Here's how the part is built. I have some questions about the finished solid (model axes, mm). Coordinates: 2 decimals unless noted, no trailing zeros. Order: outer loops, then holes, each group sorted by start corner. A loop starts at its lowest first (then second) coordinate and runs counter-clockwise, first axis right, second up. Notation, with made-up numbers: M 55.25,27 L 83.25,27 A19 ccw 83.25,52 Z; hole C -3.5,11 d2. An arc over 180 degrees is marked long. Answer as CSV lines item,"result". Start each with the question number.
```python
from build123d import *

# Parameters (mm, degrees)
ESQUISSE1_W        = 420
ESQUISSE1_H        = 560
ESQUISSE1_R        = 6.1
ESQUISSE1_R_2      = 7.5
BOSS_EXTRU_1_DEPTH = 12


with BuildPart() as part:
    # Esquisse1 → Boss.-Extru.1 (new body)
    with BuildSketch(Plane(origin=(0, 0, 0), x_dir=(1, 0, 0), z_dir=(0, 1, 0))):
        with Locations((0, -70)):
            Rectangle(ESQUISSE1_W, ESQUISSE1_H)
        with Locations(Location((-63.273726515, 173.843134845, 0), (0, 0, 270))):  # turned: the seam where the file's is
            Circle(ESQUISSE1_R, mode=Mode.SUBTRACT)
        with Locations(Location((-175, -61.5, 0), (0, 0, 270))):  # turned: the seam where the file's is
            Circle(ESQUISSE1_R_2, mode=Mode.SUBTRACT)
        with Locations(Location((110.0032143, -211.5, 0), (0, 0, 270))):  # turned: the seam where the file's is
            Circle(ESQUISSE1_R_2, mode=Mode.SUBTRACT)
        with Locations(Location((175, -61.5, 0), (0, 0, 270))):  # turned: the seam where the file's is
            Circle(ESQUISSE1_R_2, mode=Mode.SUBTRACT)
        with Locations(Location((185, 0, 0), (0, 0, 270))):  # turned: the seam where the file's is
            Circle(ESQUISSE1_R, mode=Mode.SUBTRACT)
        with Locations(Location((-109.9967857, -211.5, 0), (0, 0, 270))):  # turned: the seam where the file's is
            Circle(ESQUISSE1_R_2, mode=Mode.SUBTRACT)
        with Locations(Location((151.543128193, 106.111640725, 0), (0, 0, 90))):  # turned: the seam where the file's is
            Circle(ESQUISSE1_R, mode=Mode.SUBTRACT)
        with Locations(Location((-151.543128193, 106.111640725, 0), (0, 0, 270))):  # turned: the seam where the file's is
            Circle(ESQUISSE1_R, mode=Mode.SUBTRACT)
        with Locations(Location((-185, 0, 0), (0, 0, 90))):  # turned: the seam where the file's is
            Circle(ESQUISSE1_R, mode=Mode.SUBTRACT)
        with Locations(Location((63.273726515, 173.843134845, 0), (0, 0, 90))):  # turned: the seam where the file's is
            Circle(ESQUISSE1_R, mode=Mode.SUBTRACT)
        with Locations(Location((-145.781989417, -113.897372935, 0), (0, 0, 270))):  # turned: the seam where the file's is
            Circle(ESQUISSE1_R, mode=Mode.SUBTRACT)
        with Locations(Location((-78.184378422, -167.666940602, 0), (0, 0, 270))):  # turned: the seam where the file's is
            Circle(ESQUISSE1_R, mode=Mode.SUBTRACT)
        with Locations(Location((145.781989417, -113.897372935, 0), (0, 0, 90))):  # turned: the seam where the file's is
            Circle(ESQUISSE1_R, mode=Mode.SUBTRACT)
        with Locations(Location((78.184378422, -167.666940602, 0), (0, 0, 90))):  # turned: the seam where the file's is
            Circle(ESQUISSE1_R, mode=Mode.SUBTRACT)
        with BuildLine():
            Line((10.5, 164.654013459), (10.5, 159.154013459))
            ThreePointArc((10.5, 159.154013459), (0, -159.5), (-10.5, 159.154013459))
            Line((-10.5, 159.154013459), (-10.5, 164.654013459))
            Line((-10.5, 164.654013459), (10.5, 164.654013459))
        make_face(mode=Mode.SUBTRACT)
    extrude(amount=BOSS_EXTRU_1_DEPTH)


solid = part.part
```
1) Suppose I cut it at C-C on z = 0. Please give me the cut outline in (x, y), plus the area to 3 significant figures.
2) If we mould it in two halves opening along Z, with no side actions, what happens to faces 1 (the face through (-3, 6, 350)), 2 (the face through (145.51, 5.92, 119.99)), 3 (the face through (-3, 0, 191))? For each: released by +Z, released by -Z, zero draft, split by the parting line, or undercut.
3) Suppose I cut it at B-B on x = 0. Please give me the cut outline in (y, z), plus the area to 3 significant figures.
4) Suppose I cut it at A-A on z = 211.5. Please give me the cut outline in (x, y), plus the area to 3 significant figures.
5) I need wall thicknesses on line 1 (X direction, y = 6.25, z = 211.5); line 2 (X direction, y = 4.75, z = -178); line 3 (Z direction, x = 0, y = 9.5). Which ranges of each line are inside material? Lowest first, please. Write a range as [from, to].
6) Suppose I cut it at D-D on z = -93. Please give me the cut outline in (x, y).
Output:
1,outline,"M -210,0 L -191.1,0 L -191.1,12 L -210,12 Z; M -178.9,0 L -159.5,0 L -159.5,12 L -178.9,12 Z; M 159.5,0 L 178.9,0 L 178.9,12 L 159.5,12 Z; M 191.1,0 L 210,0 L 210,12 L 191.1,12 Z"
1,area,"919 mm²"
2,face 1,"released by +Z"
2,face 2,"undercut"
2,face 3,"zero draft"
3,outline,"M 0,-210 L 12,-210 L 12,-164.65 L 0,-164.65 Z; M 0,159.5 L 12,159.5 L 12,350 L 0,350 Z"
3,area,"2,830 mm²"
4,outline,"M -210,0 L -117.5,0 L -117.5,12 L -210,12 Z; M -102.5,0 L 102.5,0 L 102.5,12 L -102.5,12 Z; M 117.5,0 L 210,0 L 210,12 L 117.5,12 Z"
4,area,"4,680 mm²"
5,line 1,"[-210, -117.5], [-102.5, 102.5], [117.5, 210]"
5,line 2,"[-210, -67.74], [-58.81, 58.81], [67.74, 210]"
5,line 3,"[-210, -164.65], [159.5, 350]"
6,outline,"M -210,0 L -129.58,0 L -129.58,12 L -210,12 Z; M 129.58,0 L 210,0 L 210,12 L 129.58,12 Z"
